Can you work these out from the model? Positions are in its coordinate system, mm. A direction names the side the tool comes from. Coordinates: 2 decimals unless noted, no trailing zeros. Loops run counter-clockwise (first coordinate to the right, second up) from the corner with the lowest first, then second, coordinate; pieces in that order, holes last. Notation, with made-up numbers: M 38,75.25 L 67,75.25 A26 cw 67,109.25 Z; hole C 84.5,8 d3. An arc over 180 degrees is marked long. Answer as a JSON object with one key per item and string values. Group by question number.
Item 1: Which directions (+Z, -Z, +X, -X, +Y, -Y) give clear straight access to the entire face, cutting with the end or side of a thin tool? Please do faces 1 (the flat face through (53, 3, 34.5)), 2 (the cylindrical face through (54.23, 0.03, -35.75)), 3 (the flat face through (108, 3, 0)), 4 (the flat face through (55, 3, -34.5)).
Item 2: Suppose I cut it at C-C (z = -24). Write out the boundary of the cut face in (x, y).
Item 3: Suppose I cut it at B-B (x = 64). Write out the boundary of the cut face in (y, z).
Item 4: If I drill on line 1 (Y direction, x = 34, z = -1); line 2 (Z direction, x = 18.5, y = 3); line 3 (X direction, y = 2, z = 30), over which ranges is the centre line in solid material (lowest first)?
Item 5: Suppose I cut it at A-A (z = -15). Write out the boundary of the cut face in (x, y).
Item 6: I'm going to push flat-ended pins straight in: pin 1 Ø12 at (x, z) = (40, -23) entering from +Y; pin 2 Ø1.5 at (y, z) = (4, 4) entering from -X; pin 3 Ø3.5 at (y, z) = (3.5, 7) entering from +X; pin 4 Ø0.6 at (x, z) = (109, 13.5) entering from +Y. Where does each tip first touch, or does it pass through?
Autodesk Inventor part; units mm, degrees
ref_plane "YZ Plane" through (0, 0, 0) normal (1, 0, 0) x (0, 1, 0)
ref_plane "XZ Plane" through (0, 0, 0) normal (0, 1, 0) x (-1, 0, 0)
ref_plane "XY Plane" through (0, 0, 0) normal (0, 0, 1) x (1, 0, 0)
sketch "Sketch1" plane through (0, 0, 0) normal (1, 0, 0) x (0, 1, 0)
  line L0 (0, 34.5) -> (0, -34.5) construction
  line L1 (-1.25, 34.5) -> (-1.25, -34.5)
  line L2 (1.25, -34.5) -> (1.25, 34.5)
  arc A0 (1.25, 34.5) -> (-1.25, 34.5) centre (0, 34.5) ccw
  arc A1 (-1.25, -34.5) -> (1.25, -34.5) centre (0, -34.5) ccw
  line L3 (0, 0) -> (69, 0) construction
  dimension "d0" = 34.5
  dimension "d1" = 90
  dimension "d2" = 2.5
sketch "Sketch1 outline for Extrusion1" plane through (0, 0, 0) normal (1, 0, 0) x (0, 1, 0)
  arc A0 (-1.25, -34.5) -> (1.25, -34.5) centre (0, -34.5) ccw
  line L0 (-1.25, 34.5) -> (-1.25, -34.5)
  arc A1 (1.25, 34.5) -> (-1.25, 34.5) centre (0, 34.5) ccw
  line L1 (1.25, -34.5) -> (1.25, 34.5)
extrude "Extrusion1" add sketch "Sketch1 outline for Extrusion1" along normal blind 110
sketch "Sketch2" plane through (0, 1.25, 34.5) normal (0, 1, 0) x (1, 0, 0)
  line L0 (0, 34.5) -> (108, 34.5)
  line L1 (0, 34.5) -> (108, 34.5) construction
  line L2 (108, 34.5) -> (108, 69)
  line L3 (108, 34.5) -> (108, 0)
  line L4 (110, 69) -> (110, 0)
  line L5 (108, 34.5) -> (142.5, 34.5) construction
  line L6 (108, 0) -> (108, 69)
  line L7 (108, 69) -> (0, 69)
  line L8 (0, 69) -> (0, 0)
  line L9 (0, 0) -> (108, 0)
  line L10 (110, 69) -> (110, 70.25)
  line L11 (0, 69) -> (0, 0)
  dimension "d5" = 108
  dimension "d6" = 0
  dimension "d7" = 34.5
  dimension "d8" = 34.5
  dimension "d9" = 90
sketch "Sketch2 outline for Extrusion2" plane through (0, 1.25, 34.5) normal (0, 1, 0) x (1, 0, 0)
  line L0 (108, 69) -> (0, 69)
  line L1 (108, 34.5) -> (108, 69)
  line L2 (108, 0) -> (108, 34.5)
  line L3 (0, 0) -> (108, 0)
  line L4 (0, 69) -> (0, 0)
extrude "Extrusion2" add sketch "Sketch2 outline for Extrusion2" along normal blind 3
sketch "Sketch3" plane through (0, 4.25, 34.5) normal (0, 1, 0) x (1, 0, 0)
  line L0 (0, 34.5) -> (3, 34.5)
  line L1 (3, 34.5) -> (6, 34.5)
  line L2 (6, 34.5) -> (9, 34.5)
  line L3 (9, 29.5) -> (9, 39.5) construction
  line L4 (9.75, 29.5) -> (9.75, 39.5)
  line L5 (8.25, 39.5) -> (8.25, 29.5)
  arc A0 (8.25, 29.5) -> (9.75, 29.5) centre (9, 29.5) ccw
  arc A1 (9.75, 39.5) -> (8.25, 39.5) centre (9, 39.5) ccw
  line L6 (9, 34.5) -> (19, 34.5) construction
  line L7 (6, 29.5) -> (6, 39.5) construction
  line L8 (6.75, 29.5) -> (6.75, 39.5)
  line L9 (5.25, 39.5) -> (5.25, 29.5)
  arc A2 (5.25, 29.5) -> (6.75, 29.5) centre (6, 29.5) ccw
  arc A3 (6.75, 39.5) -> (5.25, 39.5) centre (6, 39.5) ccw
  line L10 (3, 29.5) -> (3, 39.5) construction
  line L11 (3.75, 29.5) -> (3.75, 39.5)
  line L12 (2.25, 39.5) -> (2.25, 29.5)
  arc A4 (2.25, 29.5) -> (3.75, 29.5) centre (3, 29.5) ccw
  arc A5 (3.75, 39.5) -> (2.25, 39.5) centre (3, 39.5) ccw
  dimension "d12" = 3
  dimension "d13" = 3
  dimension "d14" = 3
  dimension "d15" = 180
  dimension "d16" = 5
  dimension "d17" = 90
  dimension "d18" = 1.5
  dimension "d19" = 5
  dimension "d20" = 1.5
  dimension "d21" = 5
  dimension "d22" = 1.5
sketch "Sketch3 outline for Extrusion3" plane through (0, 4.25, 34.5) normal (0, 1, 0) x (1, 0, 0)
  arc A0 (9.75, 39.5) -> (8.25, 39.5) centre (9, 39.5) ccw
  line L0 (9.75, 29.5) -> (9.75, 39.5)
  arc A1 (8.25, 29.5) -> (9.75, 29.5) centre (9, 29.5) ccw
  line L1 (8.25, 39.5) -> (8.25, 29.5)
  arc A2 (5.25, 29.5) -> (6.75, 29.5) centre (6, 29.5) ccw
  line L2 (5.25, 39.5) -> (5.25, 29.5)
  arc A3 (6.75, 39.5) -> (5.25, 39.5) centre (6, 39.5) ccw
  line L3 (6.75, 29.5) -> (6.75, 39.5)
  arc A4 (2.25, 29.5) -> (3.75, 29.5) centre (3, 29.5) ccw
  line L4 (2.25, 39.5) -> (2.25, 29.5)
  arc A5 (3.75, 39.5) -> (2.25, 39.5) centre (3, 39.5) ccw
  line L5 (3.75, 29.5) -> (3.75, 39.5)
extrude "Extrusion3" add sketch "Sketch3 outline for Extrusion3" along normal blind 2 draft -45
sketch "Sketch4" plane through (0, -1.25, -34.5) normal (0, -1, 0) x (1, 0, 0)
  line L0 (0, 34.5) -> (1.5, 34.5)
  line L1 (1.5, 14.5) -> (1.5, 54.5) construction
  line L2 (6, 39.5) -> (6, 29.5)
  line L3 (2.75, 14.5) -> (2.75, 54.5)
  line L4 (0.25, 54.5) -> (0.25, 14.5)
  arc A0 (0.25, 14.5) -> (2.75, 14.5) centre (1.5, 14.5) ccw
  arc A1 (2.75, 54.5) -> (0.25, 54.5) centre (1.5, 54.5) ccw
  line L5 (1.5, 34.5) -> (41.5, 34.5) construction
  dimension "d25" = 1.5
  dimension "d26" = 20
  dimension "d27" = 90
  dimension "d28" = 2.5
sketch "Sketch4 outline for Extrusion4" plane through (0, -1.25, -34.5) normal (0, -1, 0) x (1, 0, 0)
  arc A0 (2.75, 54.5) -> (0.25, 54.5) centre (1.5, 54.5) ccw
  line L0 (2.75, 14.5) -> (2.75, 54.5)
  arc A1 (0.25, 14.5) -> (2.75, 14.5) centre (1.5, 14.5) ccw
  line L1 (0.25, 54.5) -> (0.25, 14.5)
extrude "Extrusion4" add sketch "Sketch4 outline for Extrusion4" along normal blind 2 draft -45
properties part number "Case-Top"
From the geometry:
{
 "1": {"face 1": "+Z, +X, -X, +Y", "face 2": "-Z, +X, -X", "face 3": "+Z, -Z, +X, +Y", "face 4": "-Z, +X, -X, +Y"},
 "2": {"outline": "M 0,-1.25 L 110,-1.25 L 110,1.25 L 108,1.25 L 108,4.25 L 0,4.25 Z"},
 "3": {"outline": "M -1.25,-34.5 A1.25 ccw 1.25,-34.5 L 4.25,-34.5 L 4.25,34.5 L 1.25,34.5 A1.25 ccw -1.25,34.5 Z"},
 "4": {"line 1": "-1.25 to 4.25", "line 2": "-34.5 to 34.5", "line 3": "0 to 108"},
 "5": {"outline": "M 0,-1.25 L 0.25,-1.25 L 1.5,-2.5 L 2.75,-1.25 L 110,-1.25 L 110,1.25 L 108,1.25 L 108,4.25 L 0,4.25 Z"},
 "6": {"pin 1": "y = 4.25", "pin 2": "x = 0", "pin 3": "x = 108", "pin 4": "y = 1.25"}
}
